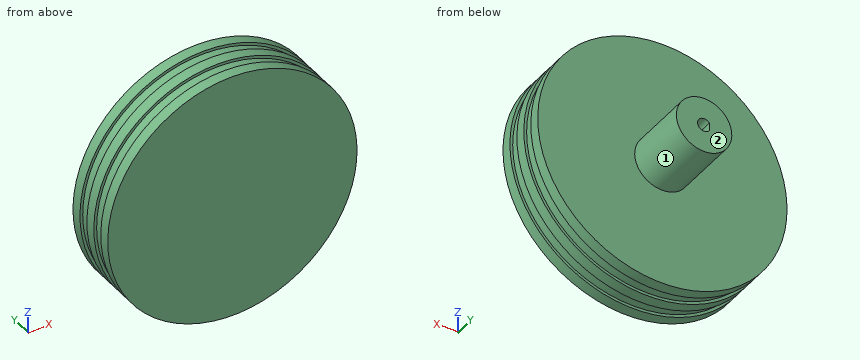
from build123d import *

# Parameters (mm, degrees)
SKETCH1_R           = 28.575
BOSS_EXTRUDE1_DEPTH = 2.54
SKETCH2_R           = 27.94
BOSS_EXTRUDE2_DEPTH = 2.54
SKETCH3_R           = 28.575
BOSS_EXTRUDE3_DEPTH = 2.54
SKETCH4_R           = 27.94
BOSS_EXTRUDE4_DEPTH = 2.54
SKETCH5_R           = 28.575
BOSS_EXTRUDE5_DEPTH = 2.54
SKETCH6_R           = 6.35
BOSS_EXTRUDE6_DEPTH = 15.24
CUT_EXTRUDE1_DEPTH  = 12.7


with BuildPart() as part:
    # Sketch1 → Boss-Extrude1 (new body)
    with BuildSketch(Plane(origin=(0, 0, 0), x_dir=(1, 0, 0), z_dir=(0, 1, 0))):
        with Locations(Location((0, 0, 0), (0, 0, 270))):
            Circle(SKETCH1_R)
    extrude(amount=BOSS_EXTRUDE1_DEPTH)

    # Sketch2 → Boss-Extrude2 (add)
    with BuildSketch(Plane(origin=(0, 2.54, 0), x_dir=(1, 0, 0), z_dir=(0, 1, 0))):
        with Locations(Location((0, 0, 0), (0, 0, 270))):
            Circle(SKETCH2_R)
    extrude(amount=BOSS_EXTRUDE2_DEPTH)

    # Sketch3 → Boss-Extrude3 (add)
    with BuildSketch(Plane(origin=(0, 5.08, 0), x_dir=(1, 0, 0), z_dir=(0, 1, 0))):
        with Locations(Location((0, 0, 0), (0, 0, 270))):
            Circle(SKETCH3_R)
    extrude(amount=BOSS_EXTRUDE3_DEPTH)

    # Sketch4 → Boss-Extrude4 (add)
    with BuildSketch(Plane(origin=(0, 7.62, 0), x_dir=(1, 0, 0), z_dir=(0, 1, 0))):
        with Locations(Location((0, 0, 0), (0, 0, 270))):
            Circle(SKETCH4_R)
    extrude(amount=BOSS_EXTRUDE4_DEPTH)

    # Sketch5 → Boss-Extrude5 (add)
    with BuildSketch(Plane(origin=(0, 10.16, 0), x_dir=(1, 0, 0), z_dir=(0, 1, 0))):
        with Locations(Location((0, 0, 0), (0, 0, 270))):
            Circle(SKETCH5_R)
    extrude(amount=BOSS_EXTRUDE5_DEPTH)

    # Sketch6 → Boss-Extrude6 (add)
    with BuildSketch(Plane(origin=(0, 12.7, 0), x_dir=(1, 0, 0), z_dir=(0, 1, 0))):
        with Locations(Location((0, 0, 0), (0, 0, 90))):
            Circle(SKETCH6_R)
    extrude(amount=BOSS_EXTRUDE6_DEPTH)

    # Sketch7 → Cut-Extrude1 (cut)
    with BuildSketch(Plane(origin=(0, 27.94, 0), x_dir=(1, 0, 0), z_dir=(0, 1, 0))):
        with BuildLine():
            Line((-1.200000076, 0.899999978), (-1.200000076, -0.899999978))
            ThreePointArc((-1.200000076, -0.899999978), (1.500000048, 0), (-1.200000076, 0.899999978))
        make_face()
    extrude(amount=-CUT_EXTRUDE1_DEPTH, mode=Mode.SUBTRACT)


solid = part.part
Read the model definition and answer for the solid it produces. Units are mm, in the model's axes. Face numbers are marked on the shaded views. A direction names the side the tool comes from. Coordinates: 2 decimals unless noted, no trailing zeros. Order: outer loops, then holes, each group sorted by start corner. A loop starts at its lowest first (then second) coordinate and runs counter-clockwise, first axis right, second up. Notation, with made-up numbers: (48, 75) - (71, 75) arc R25 cw to (71, 108) - close; hole circle Ø10 at (9, 62). An arc over 180 degrees is marked (long way). Use one line per item in the form item = value.
(1) Section D-D, the plane y = 25.75 is taken. Give the vertices of the cut face in (x, z).
Computed values:
outline = circle Ø12.7 at (0, 0); hole (-1.2, -0.9) arc R1.5 ccw (long way) to (-1.2, 0.9) - close
(2) Section B-B, the plane z = 0 is taken. Give the vertices of the cut face in (x, y) (3 decimals), then the cut area to 3 significant figures.
Computed values:
outline = (-28.575, 0) - (28.575, 0) - (28.575, 2.54) - (27.94, 2.54) - (27.94, 5.08) - (28.575, 5.08) - (28.575, 7.62) - (27.94, 7.62) - (27.94, 10.16) - (28.575, 10.16) - (28.575, 12.7) - (6.35, 12.7) - (6.35, 27.94) - (1.5, 27.94) - (1.5, 15.24) - (-1.2, 15.24) - (-1.2, 27.94) - (-6.35, 27.94) - (-6.35, 12.7) - (-28.575, 12.7) - (-28.575, 10.16) - (-27.94, 10.16) - (-27.94, 7.62) - (-28.575, 7.62) - (-28.575, 5.08) - (-27.94, 5.08) - (-27.94, 2.54) - (-28.575, 2.54) - close
area = 879 mm²
(3) Straight lines are drawn through the part: L1, parallel to X at y = 20, z = 0; L2, parallel to Y at x = -8, z = -24.5; L3, parallel to X at y = 7.5, z = -26. For each, find the intervals that lie inside material, in ascending order.
Computed values:
L1 = -6.35 to -1.2, 1.5 to 6.35
L2 = 0 to 12.7
L3 = -11.85 to 11.85
(4) Which of the six approach directions +Z, -Z, +X, -X, +Y, -Y give full straight-line access (tool end or side, diameter ignored) to the marked faces 1 and 2?
Computed values:
face_1 = +Y
face_2 = +Z, -Z, +X, -X, +Y
(5) Section C-C, the plane y = 4.25 is taken. Give the vertices of the cut face in (x, z).
Computed values:
outline = circle Ø55.88 at (0, 0)
(6) Section A-A, the plane x = 0 is taken. Give the vertices of the cut face in (y, z) (3 decimals), then the cut area to 3 significant figures.
Computed values:
outline = (0, -28.575) - (2.54, -28.575) - (2.54, -27.94) - (5.08, -27.94) - (5.08, -28.575) - (7.62, -28.575) - (7.62, -27.94) - (10.16, -27.94) - (10.16, -28.575) - (12.7, -28.575) - (12.7, -6.35) - (27.94, -6.35) - (27.94, -1.5) - (15.24, -1.5) - (15.24, 1.5) - (27.94, 1.5) - (27.94, 6.35) - (12.7, 6.35) - (12.7, 28.575) - (10.16, 28.575) - (10.16, 27.94) - (7.62, 27.94) - (7.62, 28.575) - (5.08, 28.575) - (5.08, 27.94) - (2.54, 27.94) - (2.54, 28.575) - (0, 28.575) - close
area = 875 mm²
(7) Given pin 1 Ø10 at (x, y) = (20.5, 6.5) entering from -Z; pin 2 Ø1.4 at (y, z) = (20.5, 0) entering from +X; pin 3 Ø5 at (y, z) = (22, 7.5) entering from +X, each flat-ended and moving along its own axis, determine where each tip first touches the part or whether it passes through.
Computed values:
pin_1 = -24.01
pin_2 = 6.35
pin_3 = 3.91
